from build123d import *

# Parameters (mm, degrees)
EXTRUDE_1_DEPTH     = 5
SKETCH_2_R          = 10
EXTRUDE_2_DEPTH     = 10
SKETCH_3_R          = 5
CUT_EXTRUDE_1_DEPTH = 20
SKETCH_4_W          = 30
SKETCH_4_H          = 40
EXTRUDE_3_DEPTH     = 10
SKETCH_5_R          = 15
EXTRUDE_4_DEPTH     = 25
SKETCH_6_R          = 7.5
CUT_EXTRUDE_2_DEPTH = 25
RIB_3_REACH         = 82.623
SKETCH_7_WALL_W     = 190.976004214
SKETCH_7_WALL_H     = 5


with BuildPart() as part:
    # 草图1 → 凸台-拉伸1 (new, symmetric)
    with BuildSketch(Plane.XY):
        with BuildLine():
            Line((-15, 35), (15, 35))
            Line((15, 35), (15, 13.228756555))
            ThreePointArc((15, 13.228756555), (0, -20), (-15, 13.228756555))
            Line((-15, 13.228756555), (-15, 35))
        make_face()
    extrude(amount=EXTRUDE_1_DEPTH, both=True)

    # 草图2 → 凸台-拉伸2 (add, symmetric)
    with BuildSketch(Plane.XY):
        Circle(SKETCH_2_R)
    extrude(amount=EXTRUDE_2_DEPTH, both=True)

    # 草图3 → 切除-拉伸1 (cut)
    with BuildSketch(Plane.XY.offset(10)):
        Circle(SKETCH_3_R)
    extrude(amount=-CUT_EXTRUDE_1_DEPTH, mode=Mode.SUBTRACT)

    # 草图4 → 凸台-拉伸3 (add)
    with BuildSketch(Plane(origin=(0, 35, 0), x_dir=(1, 0, 0), z_dir=(0, 1, 0))):
        with Locations((0, -15)):
            Rectangle(SKETCH_4_W, SKETCH_4_H)
    extrude(amount=EXTRUDE_3_DEPTH)

    # 草图5 → 凸台-拉伸4 (add)
    with BuildSketch(Plane.XZ.offset(-35)):
        with Locations(Location((0, 35, 0), (0, 0, 270))):
            Circle(SKETCH_5_R)
    extrude(amount=-EXTRUDE_4_DEPTH)

    # 草图6 → 切除-拉伸2 (cut)
    with BuildSketch(Plane(origin=(0, 60, 0), x_dir=(1, 0, 0), z_dir=(0, 1, 0))):
        with Locations(Location((0, -35, 0), (0, 0, 270))):
            Circle(SKETCH_6_R)
    extrude(amount=-CUT_EXTRUDE_2_DEPTH, mode=Mode.SUBTRACT)

    # 草图7 wall → 筋3 (add, up to next)
    with BuildSketch(Plane(origin=(0, 51, 7.5), x_dir=(0, 0.432731067585, 0.901523057468), z_dir=(0, -0.901523057468, 0.432731067585)), mode=Mode.PRIVATE) as rib_3_sk1:
        Rectangle(SKETCH_7_WALL_W, SKETCH_7_WALL_H)
    rib_3_tool1 = extrude(rib_3_sk1.sketch, amount=RIB_3_REACH, mode=Mode.PRIVATE) - part.part
    add(rib_3_tool1.solids().sort_by_distance((0, 51, 7.5))[0])


solid = part.part
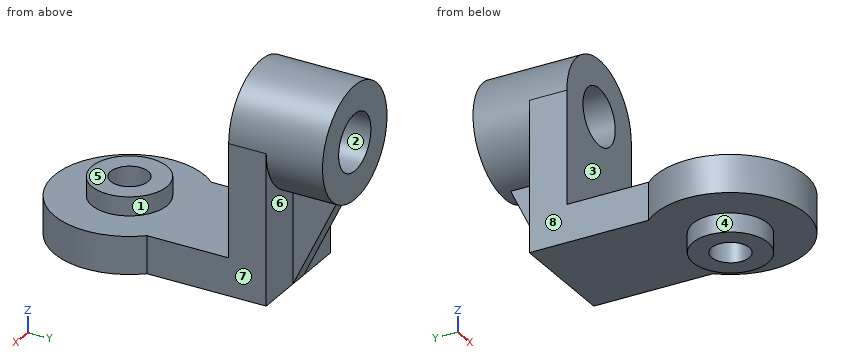
Build history of the part. All positions in model axes, mm. Face numbers are marked on the shaded views. A direction names the side the tool comes from. Round coordinates to 2 decimals unless told otherwise and drop trailing zeros. Write each loop counter-clockwise with the first axis right and the second up, starting at its lowest first coordinate (ties: lowest second). Pieces come first, ordered by that corner, then holes. Notation, with made-up numbers: M 10,40 L 56,40 A26 cw 56,57 Z; hole C 62.25,-13.75 d1. An arc over 180 degrees is marked long. Answer in a Markdown table with one row per item.
1. Mould opens along X. For the marked faces 1, 2 and 3 say: +X half, -X half, draft (parallel to the pull), parting line (faces both ways), or undercut.
Geometry check:
| item | result |
|---|---|
| face 1 | parting line |
| face 2 | undercut |
| face 3 | draft |
2. Flat gauge pins, fed straight in: P1, Ø15, axis at x = -7, z = 37, coming from the -Y side; P2, Ø1, axis at x = -8, y = 49.5, coming from the -Z side; P3, Ø1.5, axis at x = 12, y = 40.5, coming from the -Z side. Where does each tip first touch, or does it go through?
Geometry check:
| item | result |
|---|---|
| P1 | y = 35 |
| P2 | z = 22.01 |
| P3 | z = -5 |
3. Saw through at D-D (x = -12). List the corners of the cut face in (y, z), and give its area (3 significant figures).
Geometry check:
| item | result |
|---|---|
| outline | M -16,-5 L 45,-5 L 45,26 L 60,26 L 60,44 L 35,44 L 35,5 L -16,5 Z |
| area | 1,270 mm2 |
4. Saw through at C-C (y = 48). List the corners of the cut face in (x, z), and give its area (3 significant figures).
Geometry check:
| item | result |
|---|---|
| outline | M -2.5,1.25 L 2.5,1.25 L 2.5,20.21 A15 ccw long -2.5,20.21 Z; hole C 0,35 d15 |
| area | 624 mm2 |
5. Saw through at A-A (y = 0). List the corners of the cut face in (x, z).
Geometry check:
| item | result |
|---|---|
| outline | M -20,-5 L -10,-5 L -10,-10 L -5,-10 L -5,10 L -10,10 L -10,5 L -20,5 Z; M 5,-10 L 10,-10 L 10,-5 L 20,-5 L 20,5 L 10,5 L 10,10 L 5,10 Z |
6. Which spindle directions (+Z, -Z, +X, -X, +Y, -Y) get a long thin tool onto all of the face, cutting with end or side? Do the marked faces 4, 5, 6, 7 and 8. Say none if no direction does.
Geometry check:
| item | result |
|---|---|
| face 4 | -Z |
| face 5 | +Z, +X, -X, -Y |
| face 6 | -Z, +X, +Y |
| face 7 | +Z, -Z, +X, +Y |
| face 8 | +Z, -Z, -X, +Y |
7. Saw through at B-B (x = 0). List the corners of the cut face in (y, z), and give its area (4 significant figures).
Geometry check:
| item | result |
|---|---|
| outline | M -20,-5 L -10,-5 L -10,-10 L -5,-10 L -5,10 L -10,10 L -10,5 L -20,5 Z; M 5,-10 L 10,-10 L 10,-5 L 45,-5 L 57,20 L 60,20 L 60,27.5 L 35,27.5 L 35,5 L 10,5 L 10,10 L 5,10 Z; M 35,42.5 L 60,42.5 L 60,50 L 35,50 Z |
| area | 1,325 mm2 |
8. Probe L1, parallel to X at y = 43.25, z = 35; L2, parallel to Z at x = -4.5, y = 15; L3, parallel to Y at x = -12, z = 16. List the from-to ranges inside material, lowest first. Write a range as [from, to].
Geometry check:
| item | result |
|---|---|
| L1 | [-15, -7.5], [7.5, 15] |
| L2 | [-5, 5] |
| L3 | [35, 45] |
